from build123d import *

# Parameters (mm, degrees)
BOSS_EXTRUDE1_DEPTH = 60
SKETCH2_R           = 25
SKETCH2_R_2         = 15
BOSS_EXTRUDE2_DEPTH = 20
FILLET1_R           = 30
CUT_EXTRUDE1_DEPTH  = 20
CUT_EXTRUDE2_DEPTH  = 20
CUT_EXTRUDE3_START  = -14
SKETCH6_R           = 15
CUT_EXTRUDE3_DEPTH  = 14


with BuildPart() as part:
    # Sketch1 → Boss-Extrude1 (new body)
    with BuildSketch(Plane.XY):
        Polygon((0, 0), (0, 60), (10, 60), (10, 10), (110, 10), (180.64896405, 80.64896405), (188.962882852, 72.335045249), (114.1, 0), align=None)
    extrude(amount=BOSS_EXTRUDE1_DEPTH)

    # Sketch2 → Boss-Extrude2 (add)
    with BuildSketch(Plane(origin=(50, -50, 0), x_dir=(0, 0, 1), z_dir=(-0.7071067811865477, 0.7071067811865474, 0))):
        with Locations(Location((30, 154.852813742, 0), (0, 0, 90))):
            Circle(SKETCH2_R)
        with Locations(Location((30, 154.852813742, 0), (0, 0, 270))):
            Circle(SKETCH2_R_2, mode=Mode.SUBTRACT)
    extrude(amount=BOSS_EXTRUDE2_DEPTH)

    # Fillet1
    fillet1_edges = [part.edges().sort_by_distance(p)[0] for p in [
        (184.805923451, 76.49200465, 60),
        (184.805923451, 76.49200465, 0),
    ]]
    fillet(fillet1_edges, radius=FILLET1_R - 0.0001)  # a hair under: the kernel refuses the full size

    # Sketch3 → Cut-Extrude1 (cut)
    with BuildSketch(Plane(origin=(0, 10, 0), x_dir=(1, 0, 0), z_dir=(0, 1, 0))):
        with BuildLine():
            Line((50, -19.514580566), (80, -19.514580566))
            ThreePointArc((80, -19.514580566), (90, -29.514580566), (80, -39.514580566))
            Line((80, -39.514580566), (50, -39.514580566))
            ThreePointArc((50, -39.514580566), (40, -29.514580566), (50, -19.514580566))
        make_face()
    extrude(amount=-CUT_EXTRUDE1_DEPTH, mode=Mode.SUBTRACT)

    # Sketch5 → Cut-Extrude2 (cut)
    with BuildSketch(Plane.ZY):
        with BuildLine():
            Line((15, 30), (15, 130))
            ThreePointArc((15, 130), (30, 145), (45, 130))
            Line((45, 130), (45, 30))
            ThreePointArc((45, 30), (30, 15), (15, 30))
        make_face()
    extrude(amount=-CUT_EXTRUDE2_DEPTH, mode=Mode.SUBTRACT)

    # Sketch6 → Cut-Extrude3 (cut)
    with BuildSketch(Plane(origin=(50, -50, 0), x_dir=(0, 0, 1), z_dir=(-0.7071067811865477, 0.7071067811865474, 0)).offset(CUT_EXTRUDE3_START)):
        with Locations(Location((30, 154.852813742, 0), (0, 0, 270))):
            Circle(SKETCH6_R)
    extrude(amount=CUT_EXTRUDE3_DEPTH, mode=Mode.SUBTRACT)


solid = part.part
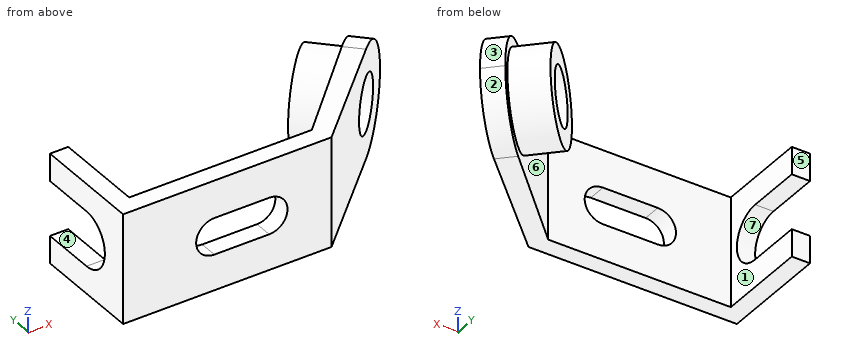
Build history of the part. All positions in model axes, mm. Face numbers are marked on the shaded views. A direction names the side the tool comes from. Coordinates: 2 decimals unless noted, no trailing zeros. Order: outer loops, then holes, each group sorted by start corner. A loop starts at its lowest first (then second) coordinate and runs counter-clockwise, first axis right, second up. Notation, with made-up numbers: M 87,29 L 107,29 A20 ccw 107,67 Z; hole C 13,-18 d4. An arc over 180 degrees is marked long. One line per question, with ' | ' between items. Start each with the question number.
Q1. Flat gauge pins, fed straight in: pin 1 Ø11 at (x, z) = (5, 51.5) entering from +Y; pin 2 Ø5 at (x, z) = (132, 35) entering from -Y; pin 3 Ø1.5 at (x, z) = (130, 25) entering from +Y. Where does each tip first touch, or does it go through?
Q2. Saw through at D-D (x = 88). List the corners of the cut face in (y, z), then the cut area to 3 significant figures.
Q3. Saw through at C-C (z = 22.5). List the corners of the cut face in (x, y), then the cut area to 3 significant figures.
Q4. Two-plate mould, pull along Z, no slides. Class the marked faces 1, 2, 3 and 4: +Z half, -Z half, draft (parallel to the pull), parting line (faces both ways), or undercut.
Q5. Saw through at B-B (y = 20.5). List the corners of the cut face in (x, z), then the cut area to 3 significant figures.
Q6. Probe L1, parallel to Z at x = 72, y = 7; L2, parallel to X at y = 35.5, z = 46; L3, parallel to Y at x = 137, z = 49. List the from-to ranges inside material, lowest first. Write a range as from..to.
Q7. 3-axis set-ups, long thin cutter, end or side, ignore diameter. For the marked faces 5, 6 and 7: which of +Z, -Z, +X, -X, +Y, -Y reach the whole face in a straight line?
Q8. Saw through at A-A (z = 41.5). List the corners of the cut face in (x, y).
Check values:
1) pin 1: stops at y = 60 | pin 2: stops at y = 14.88 | pin 3: stops at y = 59.03
2) outline: M 0,0 L 10,0 L 10,23.51 L 0,23.51 Z; M 0,35.51 L 10,35.51 L 10,60 L 0,60 Z | area: 480 mm2
3) outline: M 0,0 L 42.87,0 L 42.87,10 L 10,10 L 10,17.01 L 0,17.01 Z; M 87.13,0 L 114.1,0 L 158.1,42.52 L 136.17,64.45 L 128.49,56.78 L 142.63,42.63 L 110,10 L 87.13,10 Z; M 154.54,82.83 L 176.79,60.57 L 188.28,71.67 L 179.98,79.98 L 176.36,76.36 L 162.22,90.5 Z | area: 1,990 mm2
4) face 1: draft | face 2: -Z half | face 3: +Z half | face 4: undercut
5) outline: M 0,0 L 10,0 L 10,18.39 L 0,18.39 Z; M 0,41.61 L 10,41.61 L 10,60 L 0,60 Z; M 120.5,0 L 135.32,0 L 135.32,60 L 120.5,60 Z | area: 1,260 mm2
6) L1: z = 0..19.51, 39.51..60 | L2: x = 0..10, 135.5..150.84 | L3: y = 22.13..37, 59.02..65.28
7) face 5: +Z, -Z, -X, +Y | face 6: none | face 7: -X, +Y
8) outline: M 0,0 L 114.1,0 L 160.52,44.85 L 138.55,66.83 L 129.66,57.94 L 143.8,43.8 L 110,10 L 10,10 L 10,20.37 L 0,20.37 Z; M 152.17,80.45 L 174.38,58.24 L 187.31,70.74 L 179.03,79.03 L 175.19,75.19 L 161.05,89.34 Z
